Can you work these out from the model? Positions are in its coordinate system, mm. Face numbers are marked on the shaded views. A direction names the side the tool comes from. Coordinates: 2 decimals unless noted, no trailing zeros. Order: outer loops, then holes, each group sorted by start corner. A loop starts at its lowest first (then second) coordinate and runs counter-clockwise, first axis right, second up. Notation, with made-up numbers: (-6.5, 27.25) -> (9.5, 27.25) arc R30 cw to (9.5, 65.25) -> close; hole circle Ø2 at (-26.5, 14). An arc over 180 degrees is marked (long way). Use a Markdown table: item, result. Add a question column.
1. For pin 1 Ø2.5 at (x, z) = (2.5, -5.5) entering from -Y; pin 2 Ø6.5 at (x, z) = (37, -12) entering from -Y; pin 3 Ø7 at (x, z) = (32.5, -17.5) entering from +Y; pin 4 Ø1 at (y, z) = (-1, -15.5) entering from +X, each with a flat end and sliding along its axis, tell me the tip position at first contact or that it passes through.
2. We'd pull the mould along X, two halves only. Please class the marked faces 1, 2 and 3: pulls with the +X half, pulls with the -X half, needs draft (parallel to the pull), parting line crosses it, or undercut.
3. Suppose I cut it at A-A, the plane z = -12. List the corners of the cut face in (x, y) for me.
4. For the marked faces 4, 5 and 6, which set-ups out of +Z, -Z, +X, -X, +Y, -Y let a thin tool reach every point of the face, with its end or its side?
5. Suppose I cut it at C-C, the plane y = 4. List the corners of the cut face in (x, z) for me, then the cut area to 3 significant figures.
6. Suppose I cut it at B-B, the plane x = 2.5. List the corners of the cut face in (y, z) for me, then the cut area to 3 significant figures.
7. Suppose I cut it at D-D, the plane y = 1.5. List the corners of the cut face in (x, z) for me, then the cut area to 3 significant figures.
8. If I drill on line 1 along Z through (x, y) = (20.5, 1.75); line 2 along X through (y, z) = (0.85, -12); line 3 along Y through (x, z) = (16, -14), over which ranges is the centre line in solid material (lowest first)? Write a range as from..to.
```python
from build123d import *

# Parameters (mm, degrees)
ESBO_O1_W                = 11.5
ESBO_O1_H                = 24
ESBO_O1_R                = 2
ESBO_O1_R_2              = 3.5
ESBO_O1_W_2              = 2
RESSALTO_EXTRUS_O1_DEPTH = 2
ESBO_O1_3_R              = 2
ESBO_O1_3_R_2            = 1
RESSALTO_EXTRUS_O2_DEPTH = 5
ESBO_O1_4_W              = 2
ESBO_O1_4_H              = 24
RESSALTO_EXTRUS_O3_DEPTH = 2
CHANFRO1_SIZE            = 3
FILETE1_R                = 10


with BuildPart() as part:
    # Esboço1 → Ressalto-extrusão1 (new body)
    # profile 1 of 4: a face of its own
    with BuildSketch(Plane(origin=(0, 0, 0), x_dir=(1, 0, 0), z_dir=(0, 1, 0))):
        with Locations((5.75, 12)):
            Rectangle(ESBO_O1_W, ESBO_O1_H)
        with Locations(Location((2.5, 5.5, 0), (0, 0, 270))):
            Circle(ESBO_O1_R, mode=Mode.SUBTRACT)
        with Locations(Location((2.5, 18.5, 0), (0, 0, 270))):
            Circle(ESBO_O1_R, mode=Mode.SUBTRACT)
    # profile 2 of 4: a face of its own
    with BuildSketch(Plane(origin=(0, 0, 0), x_dir=(1, 0, 0), z_dir=(0, 1, 0))):
        with Locations((17.25, 12)):
            Rectangle(ESBO_O1_W, ESBO_O1_H)
        with Locations(Location((20.5, 5.5, 0), (0, 0, 270))):
            Circle(ESBO_O1_R, mode=Mode.SUBTRACT)
        with Locations(Location((20.5, 18.5, 0), (0, 0, 270))):
            Circle(ESBO_O1_R, mode=Mode.SUBTRACT)
    # profile 3 of 4: a face of its own
    with BuildSketch(Plane(origin=(0, 0, 0), x_dir=(1, 0, 0), z_dir=(0, 1, 0))):
        with BuildLine():
            Line((37, 24), (25, 24))
            Line((25, 24), (25, 0))
            Line((25, 0), (37, 0))
            ThreePointArc((37, 0), (49, 12), (37, 24))
        make_face()
        with Locations(Location((37, 12, 0), (0, 0, 270))):
            Circle(ESBO_O1_R_2, mode=Mode.SUBTRACT)
    # profile 4 of 4: a face of its own
    with BuildSketch(Plane(origin=(0, 0, 0), x_dir=(1, 0, 0), z_dir=(0, 1, 0))):
        with Locations((24, 12)):
            Rectangle(ESBO_O1_W_2, ESBO_O1_H)
    extrude(amount=RESSALTO_EXTRUS_O1_DEPTH)

    # Esboço1<3> → Ressalto-extrusão2 (add)
    # profile 1 of 4: a face of its own
    with BuildSketch(Plane(origin=(0, 0, 0), x_dir=(1, 0, 0), z_dir=(0, 1, 0))):
        with Locations(Location((20.5, 18.5, 0), (0, 0, 270))):
            Circle(ESBO_O1_3_R)
        with Locations(Location((20.5, 18.5, 0), (0, 0, 270))):
            Circle(ESBO_O1_3_R_2, mode=Mode.SUBTRACT)
    # profile 2 of 4: a face of its own
    with BuildSketch(Plane(origin=(0, 0, 0), x_dir=(1, 0, 0), z_dir=(0, 1, 0))):
        with Locations(Location((2.5, 18.5, 0), (0, 0, 270))):
            Circle(ESBO_O1_3_R)
        with Locations(Location((2.5, 18.5, 0), (0, 0, 270))):
            Circle(ESBO_O1_3_R_2, mode=Mode.SUBTRACT)
    # profile 3 of 4: a face of its own
    with BuildSketch(Plane(origin=(0, 0, 0), x_dir=(1, 0, 0), z_dir=(0, 1, 0))):
        with Locations(Location((2.5, 5.5, 0), (0, 0, 270))):
            Circle(ESBO_O1_3_R)
        with Locations(Location((2.5, 5.5, 0), (0, 0, 270))):
            Circle(ESBO_O1_3_R_2, mode=Mode.SUBTRACT)
    # profile 4 of 4: a face of its own
    with BuildSketch(Plane(origin=(0, 0, 0), x_dir=(1, 0, 0), z_dir=(0, 1, 0))):
        with Locations(Location((20.5, 5.5, 0), (0, 0, 270))):
            Circle(ESBO_O1_3_R)
        with Locations(Location((20.5, 5.5, 0), (0, 0, 270))):
            Circle(ESBO_O1_3_R_2, mode=Mode.SUBTRACT)
    extrude(amount=RESSALTO_EXTRUS_O2_DEPTH)

    # Esboço1<4> → Ressalto-extrusão3 (add)
    with BuildSketch(Plane(origin=(0, 0, 0), x_dir=(1, 0, 0), z_dir=(0, 1, 0))):
        with Locations((24, 12)):
            Rectangle(ESBO_O1_4_W, ESBO_O1_4_H)
    extrude(amount=-RESSALTO_EXTRUS_O3_DEPTH)

    # Chanfro1
    # the kernel refuses this chamfer: 3 mm, written as the material it adds along each edge
    with BuildSketch(Plane(origin=(20.5, 2, -18.5), x_dir=(0, 0, 1), z_dir=(-1, 0, 0))) as chanfro1_piece_1_section:
        Polygon((2 + CHANFRO1_SIZE, 0), (2, CHANFRO1_SIZE), (2, 0), align=None)
    chanfro1_piece_1 = revolve(axis=Axis((20.5, 2, -18.5), (0, 1, 0)), mode=Mode.PRIVATE)
    chanfro1_piece_1 = split(chanfro1_piece_1, bisect_by=Plane(origin=(20.5, 5, -22.010399956), z_dir=(0, -1, 0)), keep=Keep.TOP, mode=Mode.PRIVATE)
    add(chanfro1_piece_1)
    with BuildSketch(Plane(origin=(2.5, 2, -18.5), x_dir=(0, 0, 1), z_dir=(-1, 0, 0))) as chanfro1_piece_2_section:
        Polygon((2 + CHANFRO1_SIZE, 0), (2, CHANFRO1_SIZE), (2, 0), align=None)
    chanfro1_piece_2 = revolve(axis=Axis((2.5, 2, -18.5), (0, 1, 0)), mode=Mode.PRIVATE)
    chanfro1_piece_2 = split(chanfro1_piece_2, bisect_by=Plane(origin=(0, 3.427479449, -22.012332263), z_dir=(1, 0, 0)), keep=Keep.TOP, mode=Mode.PRIVATE)
    chanfro1_piece_2 = split(chanfro1_piece_2, bisect_by=Plane(origin=(2.5, 5, -22.012332263), z_dir=(0, -1, 0)), keep=Keep.TOP, mode=Mode.PRIVATE)
    add(chanfro1_piece_2)
    with BuildSketch(Plane(origin=(2.5, 2, -5.5), x_dir=(0, 0, 1), z_dir=(-1, 0, 0))) as chanfro1_piece_3_section:
        Polygon((2 + CHANFRO1_SIZE, 0), (2, CHANFRO1_SIZE), (2, 0), align=None)
    chanfro1_piece_3 = revolve(axis=Axis((2.5, 2, -5.5), (0, 1, 0)), mode=Mode.PRIVATE)
    chanfro1_piece_3 = split(chanfro1_piece_3, bisect_by=Plane(origin=(0, 3.427479449, -9.012332263), z_dir=(1, 0, 0)), keep=Keep.TOP, mode=Mode.PRIVATE)
    chanfro1_piece_3 = split(chanfro1_piece_3, bisect_by=Plane(origin=(2.5, 5, -9.012332263), z_dir=(0, -1, 0)), keep=Keep.TOP, mode=Mode.PRIVATE)
    add(chanfro1_piece_3)
    with BuildSketch(Plane(origin=(20.5, 2, -5.5), x_dir=(0, 0, 1), z_dir=(-1, 0, 0))) as chanfro1_piece_4_section:
        Polygon((2 + CHANFRO1_SIZE, 0), (2, CHANFRO1_SIZE), (2, 0), align=None)
    chanfro1_piece_4 = revolve(axis=Axis((20.5, 2, -5.5), (0, 1, 0)), mode=Mode.PRIVATE)
    chanfro1_piece_4 = split(chanfro1_piece_4, bisect_by=Plane(origin=(20.5, 5, -9.010399956), z_dir=(0, -1, 0)), keep=Keep.TOP, mode=Mode.PRIVATE)
    add(chanfro1_piece_4)

    # Filete1
    # the kernel refuses this fillet: 10 mm, written as the material it adds along each edge
    with BuildSketch(Plane(origin=(23, 0, -24), x_dir=(-1, 0, 0), z_dir=(0, 0, 1))) as filete1_piece_1_section:
        with BuildLine():
            CenterArc((6, 10), FILETE1_R, 233.130102354, 36.869897646)
            Line((0, 2), (-0.12, 1.84))
            ThreePointArc((-0.12, 1.84), (-0.2, 1), (-0.2, 0))
            Line((-0.2, 0), (0, -0.2))
            Line((0, -0.2), (6, -0.2))
            Line((6, -0.2), (6, 0))
        make_face()
    filete1_piece_1 = extrude(amount=24, mode=Mode.PRIVATE)
    filete1_piece_1 = filete1_piece_1 - Plane(origin=(20.5, -0.461272254, -5.5), x_dir=(0, 0, 1), z_dir=(0, -1, 0)) * Cylinder(1, 73, mode=Mode.PRIVATE)
    filete1_piece_1 = filete1_piece_1 - Plane(origin=(20.5, -0.461272254, -18.5), x_dir=(0, 0, 1), z_dir=(0, -1, 0)) * Cylinder(1, 73, mode=Mode.PRIVATE)
    add(filete1_piece_1)


solid = part.part
```
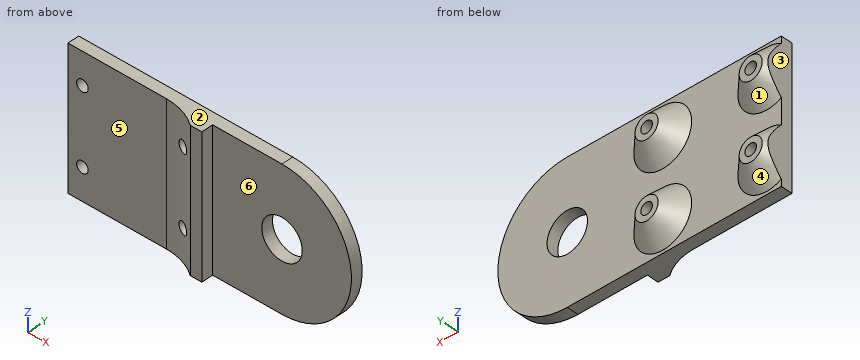
Worked out:
| question | item | result |
|---|---|---|
| 1 | pin 1 | stops at y = 0 |
| 1 | pin 2 | passes through |
| 1 | pin 3 | stops at y = 2 |
| 1 | pin 4 | stops at x = 25 |
| 2 | face 1 | undercut |
| 2 | face 2 | needs draft |
| 2 | face 3 | pulls with the -X half |
| 3 | outline | (0, 0) -> (17, 0) arc R10 cw to (23, -2) -> (25, -2) -> (25, 0) -> (33.5, 0) -> (33.5, 2) -> (0, 2) -> close; (40.5, 0) -> (49, 0) -> (49, 2) -> (40.5, 2) -> close |
| 4 | face 4 | +Y |
| 4 | face 5 | +Z, -Z, -X, -Y |
| 4 | face 6 | +Z, -Z, +X, -Y |
| 5 | outline | (0, -20.16) arc R3 ccw (long way) to (0, -16.84) -> close; (0, -7.16) arc R3 ccw (long way) to (0, -3.84) -> close; circle Ø6 at (20.5, -18.5); circle Ø6 at (20.5, -5.5); hole circle Ø2 at (2.5, -18.5); hole circle Ø2 at (2.5, -5.5); hole circle Ø2 at (20.5, -18.5); hole circle Ø2 at (20.5, -5.5) |
| 5 | area | 98.3 mm² |
| 6 | outline | (0, -24) -> (2, -24) -> (2, -23.5) -> (5, -20.5) -> (5, -19.5) -> (0, -19.5) -> close; (0, -17.5) -> (5, -17.5) -> (5, -16.5) -> (2, -13.5) -> (2, -10.5) -> (5, -7.5) -> (5, -6.5) -> (0, -6.5) -> close; (0, -4.5) -> (5, -4.5) -> (5, -3.5) -> (2, -0.5) -> (2, 0) -> (0, 0) -> close |
| 6 | area | 70.0 mm² |
| 7 | outline | (0, -24) -> (37, -24) arc R12 ccw to (37, 0) -> (0, 0) -> close; hole circle Ø2 at (2.5, -18.5); hole circle Ø2 at (2.5, -5.5); hole circle Ø2 at (20.5, -18.5); hole circle Ø2 at (20.5, -5.5); hole circle Ø7 at (37, -12) |
| 7 | area | 1,060 mm² |
| 8 | line 1 | z = -24..-19.5, -17.5..-6.5, -4.5..0 |
| 8 | line 2 | x = 0..33.5, 40.5..49 |
| 8 | line 3 | y = 0..2 |
